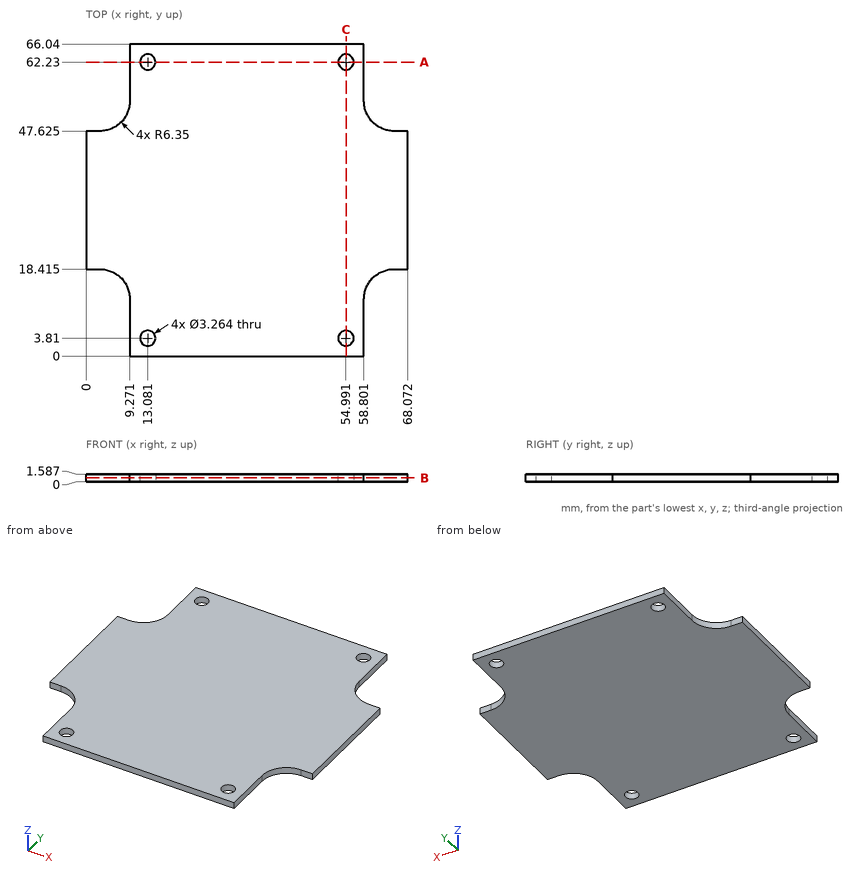
The figure shows three views and two pictorial views of one solid part (mm, origin at its lowest corner). Answer the questions. Give positions to 0.01 mm unless a question says otherwise; leave off trailing zeros. Loops run counter-clockwise (first coordinate to the right, second up) from the corner with the lowest first, then second, coordinate; pieces in that order, holes last. Notation, with made-up numbers: (75.5, 76) - (109.5, 76) arc R16 cw to (109.5, 81) - close; hole circle Ø7 at (14.25, 60.5). An arc over 180 degrees is marked (long way). Answer in a Markdown table with one row per item.
(1) Consider L1, parallel to Y at x = 14, z = 0.85; L2, parallel to X at y = 8, z = 0.75; L3, parallel to Y at x = 60.5, z = 0.9. Determine where each line is inside the solid, lowest interval first. Write a range as [from, to].
Results list:
| item | result |
|---|---|
| L1 | y = [0, 2.46], [5.16, 60.88], [63.58, 66.04] |
| L2 | x = [9.27, 58.8] |
| L3 | y = [16.39, 49.65] |
(2) Flat-ended cylindrical pins translate along their axes: pin 1 Ø2.5 at (x, y) = (13.081, 3.81) entering from +Z; pin 2 Ø0.5 at (y, z) = (3, 0.5) entering from +X; pin 3 Ø0.8 at (x, z) = (66.5, 1) entering from +Y (1 decimal); pin 4 Ø0.5 at (y, z) = (58, 1) entering from -X. Find the tip coordinate at first contact, or state that the pin passes through.
Results list:
| item | result |
|---|---|
| pin 1 | passes through |
| pin 2 | stops at x = 58.8 |
| pin 3 | stops at y = 47.6 |
| pin 4 | stops at x = 9.27 |
(3) Section A-A (y = 62.23) is taken. Give the vertices of the cut face in (x, z).
Results list:
| item | result |
|---|---|
| outline | (9.27, 0) - (11.45, 0) - (11.45, 1.59) - (9.27, 1.59) - close; (14.71, 0) - (53.36, 0) - (53.36, 1.59) - (14.71, 1.59) - close; (56.62, 0) - (58.8, 0) - (58.8, 1.59) - (56.62, 1.59) - close |
(4) Section C-C (x = 55) is taken. Give the vertices of the cut face in (y, z).
Results list:
| item | result |
|---|---|
| outline | (0, 0) - (2.18, 0) - (2.18, 1.59) - (0, 1.59) - close; (5.44, 0) - (60.6, 0) - (60.6, 1.59) - (5.44, 1.59) - close; (63.86, 0) - (66.04, 0) - (66.04, 1.59) - (63.86, 1.59) - close |
(5) Section B-B (z = 0.8) is taken. State how many separate pieces and enclosed holes the cut face has, and give its area (3 significant figures).
Results list:
| item | result |
|---|---|
| separate pieces | 1 |
| enclosed holes | 4 |
| area | 3,810 mm² |
